Geometry: final body of the model. Coordinates: model frame, mm. A direction names the side the tool comes from. Round coordinates to 2 decimals unless told otherwise and drop trailing zeros. Order: outer loops, then holes, each group sorted by start corner. A loop starts at its lowest first (then second) coordinate and runs counter-clockwise, first axis right, second up. Notation, with made-up numbers: (13.25, 80) - (67.25, 80) arc R36 ccw to (67.25, 118) - close; hole circle Ø2 at (17.25, 30). An arc over 180 degrees is marked (long way). Put each result on its own line as item: value. Start each with the question number.
(1) Section B-B (x = 0). Output: boundary loops of the cut face in (y, z) (3 decimals), and give its area (3 significant figures).
(2) Section D-D (y = -5). Output: boundary loops of the cut face in (x, z), and give its area (3 significant figures).
(3) Pin query (flat end, axial travel): P1, Ø0.7, axis at x = 0.5, z = 0, coming from the -Y side; P2, Ø1.5, axis at x = 1.5, y = 7.5, coming from the -Z side; P3, Ø2.5, axis at x = 0, y = -16.5, coming from the -Z side. Return the tip coordinate at first contact, or that it passes through.
(4) Material intervals for L1, parallel to Y at x = 0.2, z = 0.2; L2, parallel to X at y = 0.5, z = -1.7; L3, parallel to Y at x = 1.4, z = 0.6, sorted ascending. Write a range as [from, to].
(5) Section C-C (y = 15.5). Output: boundary loops of the cut face in (x, z) (3 decimals).
(6) Pull-direction query (Z, two-part tool) for faces 1 (the face through (0.02, 16.79, 1.23)), 2 (the face through (-2, 14.15, 0)), 3 (the face through (0, -14.25, 0)); classes: released by +Z, released by -Z, zero draft, split by the parting line, or undercut.
(7) Access query for faces 4 (the face through (-2, -14.15, 0)), 5 (the face through (0, -16, -0.45)), 6 (the face through (0, 16, 0.45)). Directions: +Z, -Z, +X, -X, +Y, -Y. A direction counts if a zero-diameter tool reaches every point of the face in a straight line with its end or side. Return the directions, or none.
(8) Section A-A (z = 0). Output: boundary loops of the cut face in (x, y) (3 decimals).
from build123d import *

# Parameters (mm, degrees)
F0_R     = 0.7
F1_DEPTH = 17.65
F0_R_2   = 1.475
F2_DEPTH = 15.95
F0_R_3   = 2.25
F3_DEPTH = 14.15
F6_W     = 5.524591
F6_H     = 0.9
F8_DEPTH = 3.4
F7_W     = 4.841808
F7_H     = 0.9
F9_DEPTH = 3.4


with BuildPart() as f1:
    # F0 (on Front) → F1 (new body, symmetric)
    with BuildSketch(Plane.XZ):
        Circle(F0_R)
    extrude(amount=F1_DEPTH, both=True)

    # F0 (on Front) → F2 (join, symmetric)
    with BuildSketch(Plane.XZ):
        Circle(F0_R_2)
        Circle(F0_R, mode=Mode.SUBTRACT)
    extrude(amount=F2_DEPTH, both=True)

    # F0 (on Front) → F3 (join, symmetric)
    with BuildSketch(Plane.XZ):
        Circle(F0_R_3)
        Circle(F0_R_2, mode=Mode.SUBTRACT)
    extrude(amount=F3_DEPTH, both=True)

    # F4 (on Right) → F5 (revolve)
    with BuildSketch(Plane.YZ):
        Polygon((15.95, 0.7), (17.65, 0.7), (15.95, 1.75), align=None)
        Polygon((-17.65, 0.7), (-15.95, 0.7), (-15.95, 1.75), align=None)
    revolve(axis=Axis((0, 15.95, 0), (0, -1, 0)))

    # F6 (on face) → F8 (cut)
    with BuildSketch(Plane(origin=(0, 17.65, 0), x_dir=(-1, 0, 0), z_dir=(0, 1, 0))):
        with Locations((0.045305, 0)):
            Rectangle(F6_W, F6_H)
    extrude(amount=-F8_DEPTH, mode=Mode.SUBTRACT)

    # F7 (on face) → F9 (cut)
    with BuildSketch(Plane.XZ.offset(17.65)):
        Rectangle(F7_W, F7_H)
    extrude(amount=-F9_DEPTH, mode=Mode.SUBTRACT)


solid = f1.part
Checks:
1. outline: (-17.65, -0.7) - (-15.95, -1.75) - (-15.95, -1.475) - (-14.15, -1.475) - (-14.15, -2.25) - (14.15, -2.25) - (14.15, -1.475) - (15.95, -1.475) - (15.95, -1.75) - (17.65, -0.7) - (17.65, -0.45) - (14.25, -0.45) - (14.25, 0.45) - (17.65, 0.45) - (17.65, 0.7) - (15.95, 1.75) - (15.95, 1.475) - (14.15, 1.475) - (14.15, 2.25) - (-14.15, 2.25) - (-14.15, 1.475) - (-15.95, 1.475) - (-15.95, 1.75) - (-17.65, 0.7) - (-17.65, 0.45) - (-14.25, 0.45) - (-14.25, -0.45) - (-17.65, -0.45) - close
1. area: 140 mm²
2. outline: circle Ø4.5 at (0, 0)
2. area: 15.9 mm²
3. P1: stops at y = -14.25
3. P2: stops at z = -2.12
3. P3: stops at z = -1.75
4. L1: y = [-14.25, 14.25]
4. L2: x = [-1.47, 1.47]
4. L3: y = [-16.32, -15.95], [-14.15, 14.15], [15.95, 16.32]
5. outline: (-1.405, -0.45) arc R1.475 ccw to (1.405, -0.45) - close; (-1.405, 0.45) - (1.405, 0.45) arc R1.475 ccw to start
6. face 1: released by +Z
6. face 2: zero draft
6. face 3: undercut
7. face 4: none
7. face 5: +X, -X, -Y
7. face 6: +X, -X, +Y
8. outline: (-2.25, -14.15) - (-1.475, -14.15) - (-1.475, -14.25) - (1.475, -14.25) - (1.475, -14.15) - (2.25, -14.15) - (2.25, 14.15) - (1.475, 14.15) - (1.475, 14.25) - (-1.475, 14.25) - (-1.475, 14.15) - (-2.25, 14.15) - close
